CAD build for the part. Positions are in the model's coordinates, mm. Face numbers are marked on the shaded views. Give positions to 0.01 mm unless a question says otherwise; leave off trailing zeros. Order: outer loops, then holes, each group sorted by start corner. A loop starts at its lowest first (then second) coordinate and runs counter-clockwise, first axis right, second up.
Item 1: Band-saw the part on C-C on y = 13.5. Give the cut face in (x, z).
Item 2: Band-saw the part on A-A on x = 0. Give the cut face in (y, z) (3 decimals).
Item 3: Flat gauge pins, fed straight in: P1, Ø12, axis at x = 11.5, y = 12, coming from the -Z side; P2, Ø8, axis at y = 8.5, z = 14.5, coming from the +X side; P3, Ø10, axis at x = 19.5, y = 8.5, coming from the +Z side. Where does each tip first touch, or does it go through?
Item 4: Wall check: L1, parallel to X at y = 21.45, z = 0; L2, parallel to Z at x = 0, y = 8.25; L3, parallel to Z at x = 0, y = 20. Give the ranges that are in metal, low to high.
Item 5: Band-saw the part on D-D on y = 2. Give the cut face in (x, z), plus the area to 3 significant figures.
Item 6: Band-saw the part on B-B on z = 0. Give the cut face in (x, y) (3 decimals), plus the area to 3 significant figures.
Item 7: Two-plate mould, pull along Z, no slides. Class the marked faces 1, 2 and 3: released by +Z, released by -Z, zero draft, split by the parting line, or undercut.
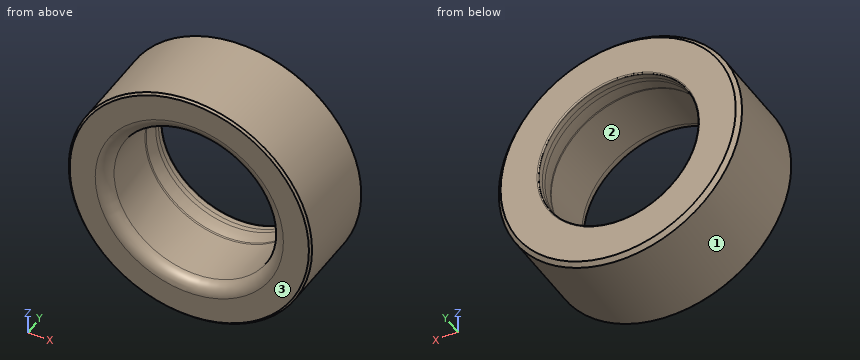
Autodesk Inventor part; units mm, degrees
ref_plane "YZ Plane" through (0, 0, 0) normal (1, 0, 0) x (0, 1, 0)
ref_plane "XZ Plane" through (0, 0, 0) normal (0, 1, 0) x (-1, 0, 0)
ref_plane "XY Plane" through (0, 0, 0) normal (0, 0, 1) x (1, 0, 0)
sketch "Náčrt1" plane through (0, 0, 0) normal (0, 0, 1) x (1, 0, 0)
  line L0 (0, 0) -> (0, 63.6053)
  line L1 (20.025, 23.5) -> (30, 23.5)
  line L2 (30, 23.5) -> (30, 0)
  line L3 (30, 0) -> (23.2, 0)
  arc A0 (20.2, 16.8138) -> (20.1389, 17.2376) centre (18.7, 16.8138) ccw
  arc A1 (19.65, 20.6279) -> (20.1389, 17.2376) centre (31.65, 20.6279) ccw
  arc A2 (20.2, 3) -> (23.2, 0) centre (23.2, 3) ccw
  line L4 (20.2, 16.8138) -> (20.2, 3)
  arc A3 (20.1, 16.9) -> (19.65, 18.2) centre (18.6153, 17.114) ccw construction
  arc A4 (19.2447, 18.8659) -> (19.65, 18.2) centre (20.6847, 19.286) ccw construction
  arc A5 (19.2447, 18.8659) -> (18.8277, 19.5429) centre (17.8047, 18.4458) ccw construction
  line L5 (13.5384, 24.4753) -> (18.8277, 19.5429) construction
  arc A6 (18.8277, 19.5429) -> (13.5384, 24.4753) centre (7.4354, 12.6284) ccw construction
  arc A7 (20.025, 23.5) -> (19.725, 23.2) centre (20.025, 23.2) ccw
  line L6 (19.65, 21.8279) -> (19.65, 20.6279)
  line L7 (19.65, 21.8279) -> (19.725, 23.0541)
  line L8 (19.65, 21.8279) -> (20.8785, 21.8279) construction
  line L9 (19.725, 23.2) -> (19.725, 23.0541)
  point P0 (19.7148, 23.5)
  dimension "d0" = 60
  dimension "d1" = 40.4
  dimension "d3" = 23.5
  dimension "d8" = 1.5
  dimension "d9" = 12
  dimension "d11" = 3
  dimension "d13" = 21.8279
  dimension "d30" = 16.8138
  dimension "d39" = 0.5
  dimension "d41" = 0.3
  dimension "d43" = 1.2
  dimension "d44" = 39.3
  dimension "d45" = 86.5
  dimension "d46" = 39.45
revolve "Rotace1" add sketch "Náčrt1" angle 360 about axis through (0, 0, 0) along (0, 1, 0)
chamfer "Zkosení1" distance 0.5 angle 45 1 edges at (-30, 0, 0)
chamfer "Zkosení3" distance 1 angle 45 1 edges at (-30, 23.5, 0)
equation "\"Rozmer_B\" = 23.5"
equation "\"Rozmer_C\" = 0"
equation "\"Rozmer_D\" = 23.5"
properties part number "NA-45-h-Crown-127" material "19 436.4"
The answers:
1. outline: circle Ø60 at (0, 0); hole circle Ø40.4 at (0, 0)
2. outline: (0, -29.5) - (0.5, -30) - (22.5, -30) - (23.5, -29) - (23.5, -20.025) arc R0.3 ccw to (23.2, -19.725) - (23.054, -19.725) - (21.828, -19.65) - (20.628, -19.65) arc R11.999 ccw to (17.238, -20.139) arc R1.501 cw to (16.814, -20.2) - (3, -20.2) arc R3 ccw to (0, -23.2) - close; (0, 23.2) arc R3 ccw to (3, 20.2) - (16.814, 20.2) arc R1.501 cw to (17.238, 20.139) arc R11.999 ccw to (20.628, 19.65) - (21.828, 19.65) - (23.054, 19.725) - (23.2, 19.725) arc R0.3 ccw to (23.5, 20.025) - (23.5, 29) - (22.5, 30) - (0.5, 30) - (0, 29.5) - close
3. P1: stops at z = -29.49
3. P2: stops at x = 28.1
3. P3: stops at z = 26.26
4. L1: x = -30 to -19.65, 19.65 to 30
4. L2: z = -30 to -20.2, 20.2 to 30
4. L3: z = -30 to -19.67, 19.67 to 30
5. outline: circle Ø60 at (0, 0); hole circle Ø40.74 at (0, 0)
5. area: 1,520 mm2
6. outline: (-30, 0.5) - (-29.5, 0) - (-23.2, 0) arc R3 ccw to (-20.2, 3) - (-20.2, 16.814) arc R1.501 cw to (-20.139, 17.238) arc R11.999 ccw to (-19.65, 20.628) - (-19.65, 21.828) - (-19.725, 23.054) - (-19.725, 23.2) arc R0.3 ccw to (-20.025, 23.5) - (-29, 23.5) - (-30, 22.5) - close; (19.65, 20.628) arc R11.999 ccw to (20.139, 17.238) arc R1.501 cw to (20.2, 16.814) - (20.2, 3) arc R3 ccw to (23.2, 0) - (29.5, 0) - (30, 0.5) - (30, 22.5) - (29, 23.5) - (20.025, 23.5) arc R0.3 ccw to (19.725, 23.2) - (19.725, 23.054) - (19.65, 21.828) - close
6. area: 461 mm2
7. face 1: split by the parting line
7. face 2: undercut
7. face 3: zero draft
